from build123d import *

# Parameters (mm, degrees)
F0_R     = 2.35
F1_DEPTH = 5
F2_R     = 3.5
F3_DEPTH = 35
F4_SIZE  = 1.016
F5_R     = 4.699
F6_DEPTH = 10
F7_R     = 0.5


with BuildPart() as f1:
    # F0 (on Top) → F1 (new body)
    with BuildSketch(Plane.XY):
        Circle(F0_R)
    extrude(amount=F1_DEPTH)

    # F2 (on face) → F3 (join)
    with BuildSketch(Plane.XY.offset(5)):
        Circle(F2_R)
    extrude(amount=F3_DEPTH)

    # F4
    f4_edges = [f1.edges().sort_by_distance(p)[0] for p in [
        (-2.35, 0, 0),
    ]]
    chamfer(f4_edges, length=F4_SIZE)

    # F5 (on face) → F6 (join)
    with BuildSketch(Plane.XY.offset(40)):
        Circle(F5_R)
    extrude(amount=-F6_DEPTH)

    # F7
    f7_edges = [f1.edges().sort_by_distance(p)[0] for p in [
        (-4.699, 0, 30),
    ]]
    fillet(f7_edges, radius=F7_R)


solid = f1.part
Geometry check sheet. Reference: the model listing, model coordinates, mm. A direction names the side the tool comes from. Give positions to 0.01 mm unless a question says otherwise; leave off trailing zeros. Loops run counter-clockwise (first coordinate to the right, second up) from the corner with the lowest first, then second, coordinate; pieces in that order, holes last. Notation, with made-up numbers: (81.5, -6) -> (111.5, -6) arc R15 ccw to (111.5, -1) -> close; hole circle Ø1 at (-38, 83). An arc over 180 degrees is marked (long way). Answer in a Markdown table with one row per item. Add a question column.
1) Material ranges on probe 1 along Z at (x, y) = (-3.5, -2.25); probe 2 along Z at (x, y) = (2, 1.5); probe 3 along Y at (x, z) = (0.25, 28), recorded low to high. Write a range as from..to.
2) Cross-section at C-C on z = 27. Record the boundary of the cut face in (x, y).
3) Set-up check for faces 1 (the face through (0, 0, 40)), 2 (the face through (-0.509, -2.294, 2.98)): record each of +Z, -Z, +X, -X, +Y, -Y from which the full face is reachable in a straight line by a thin tool's end or side.
4) Gauge pin test, flat ends, axial feed: P1, Ø2, axis at y = -2, z = 10, coming from the -X side; P2, Ø2, axis at x = 0, y = 3, coming from the -Z side; P3, Ø1, axis at x = -0.5, z = 25.5, coming from the -Y side; P4, Ø2.5, axis at x = 0.5, y = 0, coming from the -Z side. Record the tip position at first contact, or that the pin passes through.
5) Cross-section at A-A on x = 0. Record the boundary of the cut face in (y, z), and give its area (3 significant figures).
Outcome:
| question | item | result |
|---|---|---|
| 1 | probe 1 | z = 30..40 |
| 1 | probe 2 | z = 5..40 |
| 1 | probe 3 | y = -3.49..3.49 |
| 2 | outline | circle Ø7 at (0, 0) |
| 3 | face 1 | +Z, +X, -X, +Y, -Y |
| 3 | face 2 | -Z |
| 4 | P1 | stops at x = -3.35 |
| 4 | P2 | stops at z = 0.67 |
| 4 | P3 | stops at y = -3.5 |
| 4 | P4 | stops at z = 0 |
| 5 | outline | (-4.7, 30.5) arc R0.5 ccw to (-4.2, 30) -> (-3.5, 30) -> (-3.5, 5) -> (-2.35, 5) -> (-2.35, 1.02) -> (-1.33, 0) -> (1.33, 0) -> (2.35, 1.02) -> (2.35, 5) -> (3.5, 5) -> (3.5, 30) -> (4.2, 30) arc R0.5 ccw to (4.7, 30.5) -> (4.7, 40) -> (-4.7, 40) -> close |
| 5 | area | 291 mm^2 |
